from build123d import *

# Parameters (mm, degrees)
SKETCH1_R           = 11
BOSS_EXTRUDE1_DEPTH = 18.5
CUT_EXTRUDE1_DEPTH  = 4
FILLET1_R           = 1


with BuildPart() as part:
    # Sketch1 → Boss-Extrude1 (new body)
    with BuildSketch(Plane(origin=(0, 0, 0), x_dir=(1, 0, 0), z_dir=(0, 1, 0))):
        with Locations(Location((0, 0, 0), (0, 0, 270))):
            Circle(SKETCH1_R)
    extrude(amount=-BOSS_EXTRUDE1_DEPTH)

    # Sketch4 → Cut-Extrude1 (cut)
    with BuildSketch(Plane(origin=(0, 0, 0), x_dir=(1, 0, 0), z_dir=(0, 1, 0))):
        with BuildLine():
            Line((-8, -6.5), (-8, 0))
            Line((-8, 0), (-8, 6.5))
            Line((-8, 6.5), (-8.874119675, 6.5))
            ThreePointArc((-8.874119675, 6.5), (-11, 0), (-8.874119675, -6.5))
            Line((-8.874119675, -6.5), (-8, -6.5))
        make_face()
    extrude(amount=-CUT_EXTRUDE1_DEPTH, mode=Mode.SUBTRACT)

    # Fillet1
    fillet1_edges = [part.edges().sort_by_distance(p)[0] for p in [
        (9.810708435, 0, -4.974937186),
    ]]
    fillet(fillet1_edges, radius=FILLET1_R)


solid = part.part
Source: CAD feature listing. Evaluate the final solid. Frame: model axes, mm. A direction names the side the tool comes from. Give positions to 0.01 mm unless a question says otherwise; leave off trailing zeros. Write each loop counter-clockwise with the first axis right and the second up, starting at its lowest first coordinate (ties: lowest second). Pieces come first, ordered by that corner, then holes. Notation, with made-up numbers: (9.5, 62.5) -> (58.5, 62.5) arc R34 ccw to (58.5, 92.5) -> close; hole circle Ø11 at (-14.75, -7.5). An arc over 180 degrees is marked (long way). Write item = value, one per line.
Q1. First-contact query: pin 1 (2 mm diameter, centred on y = -2.5, z = 0.5, fed in from -X); pin 2 (4 mm diameter, centred on y = -13, z = -5.5, fed in from +X); pin 3 (1 mm diameter, centred on x = -8.5, y = -3, fed in from +Z). Flat tips, straight axial feed; report the tip coordinate or a pass-through.
Here are the results:
pin_1 = -8
pin_2 = 10.43
pin_3 = 7.55
Q2. Line query: line 1 (Z direction, x = 3.5, y = -9); line 2 (X direction, y = -14, z = -6.5); line 3 (Z direction, x = 6.75, y = -11.75). Output: solid intervals per line, ascending. Write a range as from..to.
Here are the results:
line_1 = -10.43..10.43
line_2 = -8.87..8.87
line_3 = -8.69..8.69
Q3. Cut plane A-A on z = 0. Return loops of the section in (x, y), then the cut area to 3 significant figures.
Here are the results:
outline = (-11, -18.5) -> (11, -18.5) -> (11, -1) arc R1 ccw to (10, 0) -> (-8, 0) -> (-8, -4) -> (-11, -4) -> close
area = 395 mm²
Q4. Reachability of faces 4 (the face through (-8.4, -2, 6.5)), 5 (the face through (1, 0, 0)) from +Z, -Z, +X, -X, +Y, -Y: full face, straight path, thin tool, end or side. Return the list, or none.
Here are the results:
face_4 = -X, +Y
face_5 = +Z, -Z, +X, -X, +Y
Q5. Mould query, pull axis Z, two halves, no side actions, for faces 1 (the face through (0, -18.5, 0)), 2 (the face through (10.906, -9.628, -1.432)), 3 (the face through (-9, -4, 0)). Classes: +Z half, -Z half, draft (parallel to the pull), parting line (faces both ways), or undercut.
Here are the results:
face_1 = draft
face_2 = parting line
face_3 = undercut
Q6. Cut plane B-B on y = -13.75. Return loops of the section in (x, z).
Here are the results:
outline = circle Ø22 at (0, 0)
